Geometry check sheet. Reference: the model listing, model coordinates, mm. Face numbers are marked on the shaded views. A direction names the side the tool comes from. Give positions to 0.01 mm unless a question says otherwise; leave off trailing zeros. Write each loop counter-clockwise with the first axis right and the second up, starting at its lowest first coordinate (ties: lowest second). Pieces come first, ordered by that corner, then holes. Notation, with made-up numbers: (53.25, -11.75) -> (86.25, -11.75) arc R27 cw to (86.25, 23.25) -> close; hole circle Ø7 at (74, 85). An arc over 180 degrees is marked (long way). One line per item, written item: value.
from build123d import *

# Parameters (mm, degrees)
F1_DEPTH = 112.7125
F2_R     = 6.35
F3_R     = 3.175
F4_T     = -1.524


with BuildPart() as f1:
    # F0 (on Right) → F1 (new body, symmetric)
    with BuildSketch(Plane.YZ):
        with BuildLine():
            ThreePointArc((-60.491874, 34.925), (-52.3875, 4.679063), (-30.245937, -17.4625))
            Line((-30.245937, -17.4625), (0, 0))
            Line((0, 0), (0, 34.925))
            ThreePointArc((0, 34.925), (-30.245937, 43.029374), (-60.491874, 34.925))
        make_face()
    extrude(amount=F1_DEPTH, both=True)

    # F2
    f2_edges = [f1.edges().sort_by_distance(p)[0] for p in [
        (0, -60.491874, 34.925),
        (0, 0, 0),
    ]]
    fillet(f2_edges, radius=F2_R)

    # F3
    f3_edges = [f1.edges().sort_by_distance(p)[0] for p in [
        (0, 0, 34.925),
        (0, -30.245937, -17.4625),
    ]]
    fillet(f3_edges, radius=F3_R)

    # F4
    f4_openings = [f1.faces().sort_by_distance(p)[0] for p in [
        (-112.7125, -28.547695, 16.482019),
        (112.7125, -28.547695, 16.482019),
    ]]
    offset(amount=F4_T, openings=f4_openings)


solid = f1.part
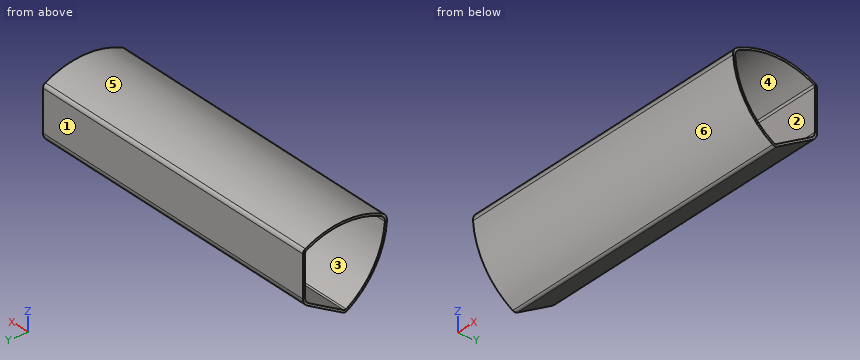
1) Scan lines: probe 1 along Z at (x, y) = (85, -30.5); probe 2 along Y at (x, z) = (60, -0.5); probe 3 along Y at (x, z) = (-19.5, -12). Record each from-to range of solid material in increasing order.
Verdict:
probe 1: -16.94 to -15.41, 41.5 to 43.03
probe 2: -49.03 to -47.14, -3.91 to -1.56
probe 3: -38.17 to -35.71, -23.83 to -20.78
2) Sectioned sample at B-B on y = -17. Record the cut outline in (x, z).
Verdict:
outline: (-112.71, -9.81) -> (112.71, -9.81) -> (112.71, -8.06) -> (-112.71, -8.06) -> close; (-112.71, 40) -> (112.71, 40) -> (112.71, 41.56) -> (-112.71, 41.56) -> close
3) Mould release check, pull along Z, two halves, no side actions. Record for the marked faces 3, 4, 5 and 6: released by +Z, released by -Z, zero draft, split by the parting line, or undercut.
Verdict:
face 3: undercut
face 4: undercut
face 5: released by +Z
face 6: released by -Z
4) Tool access check on the marked faces 1 and 2. Record the directions out of +Z, -Z, +X, -X, +Y, -Y that give a thin tool (end or side, any length) a straight path to the whole face; none if there is none.
Verdict:
face 1: +Z, -Z, +X, -X, +Y
face 2: +X, -X
5) Sectioned sample at A-A on z = 16.5. Record the cut outline in (x, y).
Verdict:
outline: (-112.71, -57.62) -> (112.71, -57.62) -> (112.71, -56.02) -> (-112.71, -56.02) -> close; (-112.71, -1.52) -> (112.71, -1.52) -> (112.71, 0) -> (-112.71, 0) -> close
6) Depth check by flat-ended pin: pin 1 Ø6 at (x, y) = (-51, -8) entering from +Z; pin 2 Ø10 at (x, z) = (-52.5, 32.5) entering from -Y; pin 3 Ø4 at (x, z) = (58.5, 36.5) entering from -Y; pin 4 Ø3 at (x, y) = (-31, -42) entering from -Z. Enter the tip coordinate at first touch or a pass-through.
Verdict:
pin 1: z = 39.89
pin 2: y = -60.36
pin 3: y = -59.43
pin 4: z = -10.01
